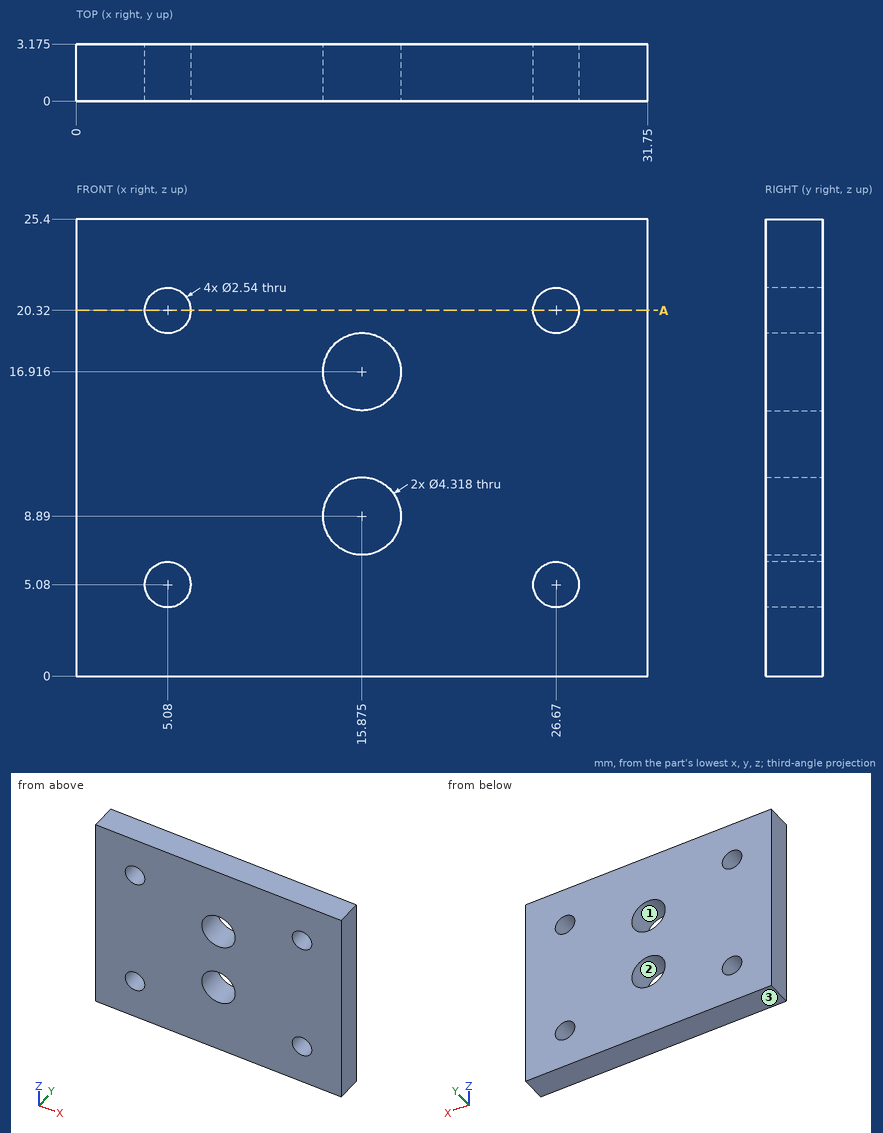
Job drawing, mm, ordinate dimensions from the low corner. One solid piece. Round coordinates to 2 decimals unless told otherwise and drop trailing zeros.
(1) Wall check: line 1 along X through (y, z) = (2.45, 5); line 2 along Z through (x, y) = (15.5, 1.65); line 3 along Z through (x, y) = (14, 2.7) (1 decimal). Give the ranges that are in metal, low to high.
(2) Cut at A-A (z = 20.32). State how many separate pieces and enclosed holes the cut face has.
(3) Two-plate mould, pull along X, no slides. Class the marked faces 1, 2 and 3: +X half, -X half, draft (parallel to the pull), parting line (faces both ways), or undercut.
Findings below:
1. line 1: x = 0 to 3.81, 6.35 to 25.4, 27.94 to 31.75
1. line 2: z = 0 to 6.76, 11.02 to 14.79, 19.04 to 25.4
1. line 3: z = 0 to 7.8, 10 to 15.8, 18 to 25.4
2. separate pieces: 3
2. enclosed holes: 0
3. face 1: undercut
3. face 2: undercut
3. face 3: draft
